```python
from build123d import *

# Parameters (mm, degrees)
BOSS_EXTRU_1_DEPTH      = 42
ESQUISSE3_W             = 35
ESQUISSE3_H             = 32
ENL_V_MAT_EXTRU_2_DEPTH = 8
ESQUISSE2_R             = 1.5
ENL_V_MAT_EXTRU_3_DEPTH = 43
CONG_1_R                = 10


with BuildPart() as part:
    # Esquisse1 → Boss.-Extru.1 (new body)
    with BuildSketch(Plane.XY):
        Polygon((0, 7), (0, 27), (-10, 27), (-10, 0), (0, 0), (35, 0), (35, 7), align=None)
    extrude(amount=BOSS_EXTRU_1_DEPTH)

    # Esquisse3 → Enlèv. mat.-Extru.2 (cut, through all)
    with BuildSketch(Plane(origin=(0, 7, 0), x_dir=(1, 0, 0), z_dir=(0, 1, 0))):
        with Locations((17.5, -21)):
            Rectangle(ESQUISSE3_W, ESQUISSE3_H)
    extrude(amount=-ENL_V_MAT_EXTRU_2_DEPTH, mode=Mode.SUBTRACT)

    # Esquisse2 → Enlèv. mat.-Extru.3 (cut, through all)
    with BuildSketch(Plane.XY.offset(42)):
        with Locations((31.75, 3.5)):
            Circle(ESQUISSE2_R)
        with Locations((23.75, 3.5)):
            Circle(ESQUISSE2_R)
        with Locations((15.75, 3.5)):
            Circle(ESQUISSE2_R)
        with Locations((7.75, 3.5)):
            Circle(ESQUISSE2_R)
    extrude(amount=-ENL_V_MAT_EXTRU_3_DEPTH, mode=Mode.SUBTRACT)

    # Congé1
    cong_1_edges = [part.edges().sort_by_distance(p)[0] for p in [
        (0, 7, 39.5),
        (0, 7, 2.5),
    ]]
    fillet(cong_1_edges, radius=CONG_1_R)


solid = part.part
```
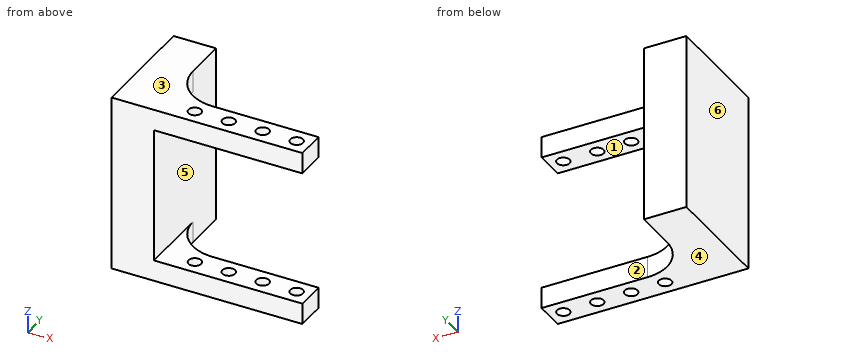
Verification items for the finished model (mm, model axes). Face numbers are marked on the shaded views. A direction names the side the tool comes from. Round coordinates to 2 decimals unless told otherwise and drop trailing zeros. Order: outer loops, then holes, each group sorted by start corner. A loop starts at its lowest first (then second) coordinate and runs counter-clockwise, first axis right, second up. Notation, with made-up numbers: (57.25, -14) -> (78.25, -14) arc R21 ccw to (78.25, -5) -> close; hole circle Ø4 at (-21, 68). An arc over 180 degrees is marked (long way). Put each result on its own line as item: value. Start each with the question number.
(1) Depth check by flat-ended pin: pin 1 Ø5 at (y, z) = (22.5, 32.5) entering from +X; pin 2 Ø13.5 at (y, z) = (15, 10.5) entering from +X; pin 3 Ø1.5 at (x, z) = (18, 3) entering from +Y. Enter the tip coordinate at first touch or a pass-through.
(2) Tool access check on the marked faces 1, 2 and 3. Record the directions out of +Z, -Z, +X, -X, +Y, -Y that give a thin tool (end or side, any length) a straight path to the whole face; none if there is none.
(3) Section check A-A (x = 31.75). Enter the section's corners in (y, z), then the cut area to 3 significant figures.
(4) Section check D-D (z = 29.5). Enter the section's corners in (x, y).
(5) Section check B-B (z = 38). Enter the section's corners in (x, y), then the cut area to 3 significant figures.
(6) Draft check along X on the marked faces 4, 5 and 6. Enter one of: +X half, -X half, draft (parallel to the pull), parting line (faces both ways), or undercut.
(7) Material ranges on line 1 along Y through (x, z) = (15.75, 1.9); line 2 along Z through (x, y) = (25.5, 5.5); line 3 along X through (y, z) = (17.25, 12), recorded low to high.
Completed:
1. pin 1: stops at x = 0
1. pin 2: stops at x = 1.94
1. pin 3: stops at y = 7
2. face 1: +X, +Y, -Y
2. face 2: +Z, -Z, +X, +Y
2. face 3: +Z, +X, -X, +Y, -Y
3. outline: (0, 0) -> (2, 0) -> (2, 5) -> (0, 5) -> close; (0, 37) -> (2, 37) -> (2, 42) -> (0, 42) -> close; (5, 0) -> (7, 0) -> (7, 5) -> (5, 5) -> close; (5, 37) -> (7, 37) -> (7, 42) -> (5, 42) -> close
3. area: 40.0 mm2
4. outline: (-10, 0) -> (0, 0) -> (0, 27) -> (-10, 27) -> close
5. outline: (-10, 0) -> (35, 0) -> (35, 7) -> (10, 7) arc R10 cw to (0, 17) -> (0, 27) -> (-10, 27) -> close; hole circle Ø3 at (7.75, 3.5); hole circle Ø3 at (15.75, 3.5); hole circle Ø3 at (23.75, 3.5); hole circle Ø3 at (31.75, 3.5)
5. area: 508 mm2
6. face 4: draft
6. face 5: +X half
6. face 6: -X half
7. line 1: y = 0 to 2, 5 to 7
7. line 2: z = 0 to 5, 37 to 42
7. line 3: x = -10 to 0
